For this review, take the finished solid that the model builds, in its own axes (mm). Face numbers are marked on the shaded views. A direction names the side the tool comes from. Give positions to 0.01 mm unless a question says otherwise; leave off trailing zeros. Loops run counter-clockwise (first coordinate to the right, second up) from the corner with the lowest first, then second, coordinate; pieces in that order, holes last.
```python
from build123d import *

# Parameters (mm, degrees)
SKETCH026_R         = 20
PAD026_DEPTH        = 9
SKETCH025_R         = 20
PAD025_DEPTH        = 1
REVOLUTION001_ANGLE = -360


with BuildPart() as screwshouldercutout:
    # Sketch026 → Pad026 (new body)
    with BuildSketch(Plane.XY):
        Circle(SKETCH026_R)
        with BuildLine():
            ThreePointArc((-2.65165, -5.833631), (-2.65165, -2.65165), (-5.833631, -2.65165))
            Line((-5.833631, -2.65165), (-12.077589, -8.895608))
            ThreePointArc((-12.077589, 8.895608), (-15, 0), (-12.077589, -8.895608))
            Line((-7.247845, 4.065864), (-12.077589, 8.895608))
            ThreePointArc((-7.247845, 4.065864), (-4.065864, 4.065864), (-4.065864, 7.247845))
            Line((-4.065864, 7.247845), (-8.895608, 12.077589))
            ThreePointArc((8.895608, 12.077589), (0, 15), (-8.895608, 12.077589))
            Line((2.65165, 5.833631), (8.895608, 12.077589))
            ThreePointArc((2.65165, 5.833631), (2.65165, 2.65165), (5.833631, 2.65165))
            Line((5.833631, 2.65165), (12.077589, 8.895608))
            ThreePointArc((12.077589, -8.895608), (15, 0), (12.077589, 8.895608))
            Line((7.247845, -4.065864), (12.077589, -8.895608))
            ThreePointArc((7.247845, -4.065864), (4.065864, -4.065864), (4.065864, -7.247845))
            Line((4.065864, -7.247845), (8.895608, -12.077589))
            ThreePointArc((-8.895608, -12.077589), (0, -15), (8.895608, -12.077589))
            Line((-2.65165, -5.833631), (-8.895608, -12.077589))
        make_face(mode=Mode.SUBTRACT)
    extrude(amount=-PAD026_DEPTH)


with BuildPart() as screwshouldercutout_1:
    # Body027 placement: moved
    add(screwshouldercutout.part.moved(Location((0, 0, -1))))


with BuildPart() as screwmountcutout:
    # Sketch025 → Pad025 (new body)
    with BuildSketch(Plane.XY):
        Circle(SKETCH025_R)
        with BuildLine():
            ThreePointArc((-2.65165, -5.833631), (-2.65165, -2.65165), (-5.833631, -2.65165))
            Line((-5.833631, -2.65165), (-12.077589, -8.895608))
            ThreePointArc((-11.453593, 9.685826), (-14.991549, 0.503442), (-12.077589, -8.895608))
            Line((-6.540738, 4.772971), (-11.453593, 9.685826))
            ThreePointArc((-6.540738, 4.772971), (-4.772971, 4.772971), (-4.772971, 6.540738))
            Line((-4.772971, 6.540738), (-9.685826, 11.453593))
            ThreePointArc((8.895608, 12.077589), (-0.503442, 14.991549), (-9.685826, 11.453593))
            Line((2.65165, 5.833631), (8.895608, 12.077589))
            ThreePointArc((2.65165, 5.833631), (2.65165, 2.65165), (5.833631, 2.65165))
            Line((5.833631, 2.65165), (12.077589, 8.895608))
            ThreePointArc((11.453593, -9.685826), (14.991549, -0.503442), (12.077589, 8.895608))
            Line((6.540738, -4.772971), (11.453593, -9.685826))
            ThreePointArc((6.540738, -4.772971), (4.772971, -4.772971), (4.772971, -6.540738))
            Line((4.772971, -6.540738), (9.685826, -11.453593))
            ThreePointArc((-8.895608, -12.077589), (0.503442, -14.991549), (9.685826, -11.453593))
            Line((-2.65165, -5.833631), (-8.895608, -12.077589))
        make_face(mode=Mode.SUBTRACT)
    extrude(amount=-PAD025_DEPTH)


with BuildPart() as cone001:
    # Sketch027 → Revolution001 (revolve, symmetric)
    with BuildSketch(Plane.YZ) as revolution001_sk:
        with BuildLine():
            Line((0, 0), (9.5, 0))
            Line((9.5, 0), (9.5, -1))
            add(Edge.make_bspline(
                [(0, -3.25), (9.5, -3.25), (9.5, -1)],
                knots=[4.712389, 4.712389, 4.712389, 6.283185, 6.283185, 6.283185], degree=2, weights=[1, 0.707107, 1]))
            Line((0, -3.25), (0, 0))
        make_face()
    revolve(axis=Axis((0, 0, 0), (0, 0, 1)), revolution_arc=REVOLUTION001_ANGLE / 2)
    revolve(revolution001_sk.sketch, axis=Axis((0, 0, 0), (0, 0, -1)), revolution_arc=REVOLUTION001_ANGLE / 2)

    # Boolean005: cut ScrewShoulderCutout, ScrewMountCutout
    add(screwshouldercutout_1.part, mode=Mode.SUBTRACT)
    add(screwmountcutout.part, mode=Mode.SUBTRACT)


solid = cone001.part
```
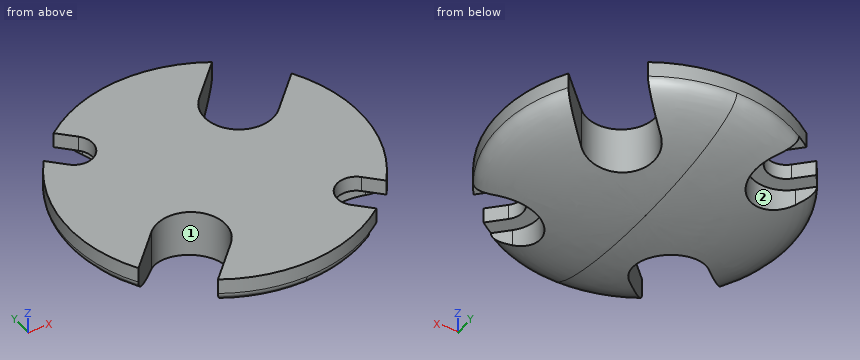
Q1. For probe 1 along Y at (x, z) = (-4.25, -1.7); probe 2 along X at (y, z) = (3, -0.3); probe 3 along Y at (x, z) = (2.25, -0.7), list the stretches that pass through material, from the lowest coordinate up.
Answers:
probe 1: y = -7.97 to -7.43, -1.99 to 3.9, 7.43 to 7.97
probe 2: x = -9.01 to 2.37, 6.18 to 9.01
probe 3: y = -9.23 to 3.2, 5.29 to 9.23
Q2. Consider section A-A on z = -0.4. Give the boundary of the cut face in (x, y), plus the area to 3 significant figures.
Answers:
outline: (-8.12, -4.94) - (-5.83, -2.65) arc R2.25 cw to (-2.65, -5.83) - (-4.94, -8.12) arc R9.5 ccw to (5.78, -7.54) - (4.77, -6.54) arc R1.25 cw to (6.54, -4.77) - (7.54, -5.78) arc R9.5 ccw to (8.12, 4.94) - (5.83, 2.65) arc R2.25 cw to (2.65, 5.83) - (4.94, 8.12) arc R9.5 ccw to (-5.78, 7.54) - (-4.77, 6.54) arc R1.25 cw to (-6.54, 4.77) - (-7.54, 5.78) arc R9.5 ccw to start
area: 225 mm2
Q3. Machinability: for the marked faces 1 and 2, which of the approach directions +Z, -Z, +X, -X, +Y, -Y give a long, thin tool a straight path to every point of the face, cutting with its end or side? Answer none if there is none.
Answers:
face 1: +Z, -Z
face 2: -Z
Q4. For pin 1 Ø6 at (x, y) = (-3.5, -7) entering from -Z; pin 2 Ø1.4 at (x, y) = (-6, 5.5) entering from -Z; pin 3 Ø3 at (x, y) = (5.5, 1.5) entering from -Z; pin 4 Ø1.4 at (x, y) = (5, -7) entering from -Z, all flat-tipped, find the tip position at first contact; note any pin that passes through.
Answers:
pin 1: stops at z = -2.94
pin 2: passes through
pin 3: stops at z = -3.02
pin 4: stops at z = -1
